from build123d import *

# Parameters (mm, degrees)
BOSS_EXTRUDE1_DEPTH = 123
SKETCH2_R           = 12
BOSS_EXTRUDE2_DEPTH = 58
BOSS_EXTRUDE3_START = 58
SKETCH3_R           = 12
BOSS_EXTRUDE3_DEPTH = 58


with BuildPart() as part:
    # Sketch1 → Boss-Extrude1 (new body)
    with BuildSketch(Plane.XY):
        Polygon((-9, 15.15359655), (9, 15.15359655), (18.714345659, 0), (9, -15.15359655), (-9, -15.15359655), (-18.714345659, 0), align=None)
    extrude(amount=BOSS_EXTRUDE1_DEPTH)

    # Sketch2 → Boss-Extrude2 (add)
    with BuildSketch(Plane(origin=(0, 0, 0), x_dir=(-1, 0, 0), z_dir=(0, 0, -1))):
        with Locations(Location((0, 0, 0), (0, 0, 180))):
            Circle(SKETCH2_R)
    extrude(amount=BOSS_EXTRUDE2_DEPTH)

    # Sketch3 → Boss-Extrude3 (add)
    with BuildSketch(Plane.XY.offset(123).offset(BOSS_EXTRUDE3_START)):
        Circle(SKETCH3_R)
    extrude(amount=-BOSS_EXTRUDE3_DEPTH)


solid = part.part
Can you work these out from the model? Positions are in its coordinate system, mm. A direction names the side the tool comes from. Give positions to 0.01 mm unless a question says otherwise; leave off trailing zeros. Write each loop counter-clockwise with the first axis right and the second up, starting at its lowest first coordinate (ties: lowest second). Pieces come first, ordered by that corner, then holes. Notation, with made-up numbers: M 35.25,67.25 L 83.25,67.25 A15 cw 83.25,91.25 Z; hole C 89,75 d11. An arc over 180 degrees is marked long. Answer in a Markdown table with one row per item. Add a question column.
Item 1: Imagine slicing it at C-C, the plane y = -6.5. Write out the boundary of the cut face in (x, z).
Item 2: Imagine slicing it at D-D, the plane z = -16.5. Write out the boundary of the cut face in (x, y), plus the area to 3 significant figures.
Item 3: Imagine slicing it at A-A, the plane x = -7. Write out the boundary of the cut face in (y, z), plus the area to 3 significant figures.
Item 4: For pin 1 Ø10 at (y, z) = (3.5, 38) entering from +X; pin 2 Ø8 at (y, z) = (-4, -5.5) entering from +X; pin 3 Ø6 at (x, z) = (3.5, -23) entering from -Y, each with a flat end and sliding along its axis, tell me the tip position at first contact or that it passes through.
Item 5: Please list where these lines run through material, in increasing order: L1, parallel to Z at x = -7, y = -13; L2, parallel to X at y = -10.5, z = 68; L3, parallel to Y at x = 0, z = -46.
Item 6: Imagine slicing it at B-B, the plane z = 114. Write out the boundary of the cut face in (x, y), plus the area to 3 significant figures.
Item 7: On a 3-axis mill with a long thin cutter (end or side, diameter ignored), from which of +Z, -Z, +X, -X, +Y, -Y can I reach the whole of each face in a straight line? I mean faces 1 (the flat face through (0, 15.154, 61)), 2 (the flat face through (-7, 10, 0)), 3 (the flat face through (-7, 10, 123)). Say none if no direction works.
Evaluation:
| question | item | result |
|---|---|---|
| 1 | outline | M -14.55,0 L -10.09,0 L -10.09,-58 L 10.09,-58 L 10.09,0 L 14.55,0 L 14.55,123 L 10.09,123 L 10.09,181 L -10.09,181 L -10.09,123 L -14.55,123 Z |
| 2 | outline | C 0,0 d24 |
| 2 | area | 452 mm² |
| 3 | outline | M -15.15,0 L -9.75,0 L -9.75,-58 L 9.75,-58 L 9.75,0 L 15.15,0 L 15.15,123 L 9.75,123 L 9.75,181 L -9.75,181 L -9.75,123 L -15.15,123 Z |
| 3 | area | 5,990 mm² |
| 4 | pin 1 | stops at x = 18.71 |
| 4 | pin 2 | stops at x = 12 |
| 4 | pin 3 | stops at y = -11.99 |
| 5 | L1 | z = 0 to 123 |
| 5 | L2 | x = -11.98 to 11.98 |
| 5 | L3 | y = -12 to 12 |
| 6 | outline | M -18.71,0 L -9,-15.15 L 9,-15.15 L 18.71,0 L 9,15.15 L -9,15.15 Z |
| 6 | area | 840 mm² |
| 7 | face 1 | +Z, -Z, +X, -X, +Y |
| 7 | face 2 | -Z |
| 7 | face 3 | +Z |
